```python
from build123d import *

# Parameters (mm, degrees)
F0_W     = 155
F0_H     = 130.75
F1_DEPTH = 3
F2_W     = 113.37
F2_H     = 92
F3_DEPTH = 25
F4_W     = 119.37
F4_H     = 98
F5_DEPTH = 25
F6_R     = 1.5
F7_DEPTH = 2
F8_W     = 155
F8_H     = 3
F9_DEPTH = 11.5


with BuildPart() as f1:
    # F0 (on Front) → F1 (new body)
    with BuildSketch(Plane.XZ):
        Rectangle(F0_W, F0_H)
    extrude(amount=F1_DEPTH)

    # F2 (on face) → F3 (cut)
    with BuildSketch(Plane(origin=(0, 0, 0), x_dir=(-1, 0, 0), z_dir=(0, 1, 0))):
        with Locations((7.5, 3.68)):
            Rectangle(F2_W, F2_H)
    extrude(amount=-F3_DEPTH, mode=Mode.SUBTRACT)

    # F4 (on face) → F5 (cut)
    with BuildSketch(Plane.XZ.offset(3)):
        with Locations((-7.5, 3.68)):
            Rectangle(F4_W, F4_H)
    extrude(amount=-F5_DEPTH, mode=Mode.SUBTRACT)

    # F6 (on face) → F7 (cut)
    with BuildSketch(Plane(origin=(0, 0, 0), x_dir=(-1, 0, 0), z_dir=(0, 1, 0))):
        with Locations((-55.685, 56.18)):
            Circle(F6_R)
        with Locations((70.685, 56.18)):
            Circle(F6_R)
        with Locations((70.685, -48.82)):
            Circle(F6_R)
        with Locations((-55.685, -48.82)):
            Circle(F6_R)
        with Locations((7.5, -48.82)):
            Circle(F6_R)
        with Locations((-55.685, 3.68)):
            Circle(F6_R)
        with Locations((70.685, 3.68)):
            Circle(F6_R)
        with Locations((7.5, 56.18)):
            Circle(F6_R)
    extrude(amount=-F7_DEPTH, mode=Mode.SUBTRACT)

    # F8 (on face) → F9 (join)
    with BuildSketch(Plane.XY.offset(65.375)):
        with Locations((0, -1.5)):
            Rectangle(F8_W, F8_H)
    extrude(amount=F9_DEPTH)


solid = f1.part
```
Work out the finished part from the listing and answer in its coordinate system (mm). Coordinates: 2 decimals unless noted, no trailing zeros. Loops run counter-clockwise (first coordinate to the right, second up) from the corner with the lowest first, then second, coordinate; pieces in that order, holes last. Notation, with made-up numbers: (47.25, 78.25) - (61.25, 78.25) arc R21 ccw to (61.25, 105.25) - close; hole circle Ø1 at (59.25, 0). An arc over 180 degrees is marked (long way). Use a Markdown table: item, result.
Item 1: Given pin 1 Ø1.5 at (x, z) = (56, -48.5) entering from +Y, flat-ended and moving along its own axis, determine where the tip first touches the part or whether it passes through.
Evaluation:
| item | result |
|---|---|
| pin 1 | stops at y = -2 |
Item 2: Find section C-C, the plane x = -13.5. Determine the outline of the cut face in (y, z) (3 decimals), and give its area (3 significant figures).
Evaluation:
| item | result |
|---|---|
| outline | (-3, -65.375) - (0, -65.375) - (0, -45.32) - (-3, -45.32) - close; (-3, 52.68) - (0, 52.68) - (0, 76.875) - (-3, 76.875) - close |
| area | 133 mm2 |
Item 3: Consider probe 1 along Z at (x, y) = (-7.5, -0.9) (3 decimals); probe 2 along Z at (x, y) = (-9.5, -2.4) (3 decimals); probe 3 along X at (y, z) = (-0.6, 46) (3 decimals). Determine where each line is inside the solid, lowest interval first. Write a range as from..to.
Evaluation:
| item | result |
|---|---|
| probe 1 | z = -65.375..-50.32, -47.32..-45.32, 52.68..54.68, 57.68..76.875 |
| probe 2 | z = -65.375..-45.32, 52.68..76.875 |
| probe 3 | x = -77.5..-67.185, 52.185..77.5 |
Item 4: Find section B-B, the plane z = -22. Determine the outline of the cut face in (x, y) (3 decimals).
Evaluation:
| item | result |
|---|---|
| outline | (-77.5, -3) - (-67.185, -3) - (-67.185, 0) - (-77.5, 0) - close; (52.185, -3) - (77.5, -3) - (77.5, 0) - (52.185, 0) - close |
Item 5: Find section A-A, the plane y = -0.85. State how many separate pieces and enclosed holes the cut face has, and give its area (3 significant figures).
Evaluation:
| item | result |
|---|---|
| separate pieces | 1 |
| enclosed holes | 9 |
| area | 10,300 mm2 |
